Part print with two shaded views. Sizes in mm from the minimum x, y, z corner. A direction names the side the tool comes from. Round coordinates to 2 decimals unless told otherwise and drop trailing zeros. Loops run counter-clockwise (first coordinate to the right, second up) from the corner with the lowest first, then second, coordinate; pieces in that order, holes last. Notation, with made-up numbers: (-33, 73.25) - (8, 73.25) arc R25 cw to (8, 106.25) - close; hole circle Ø6 at (-30, 61). An arc over 180 degrees is marked (long way). Put each result on its own line as item: value. Start each with the question number.
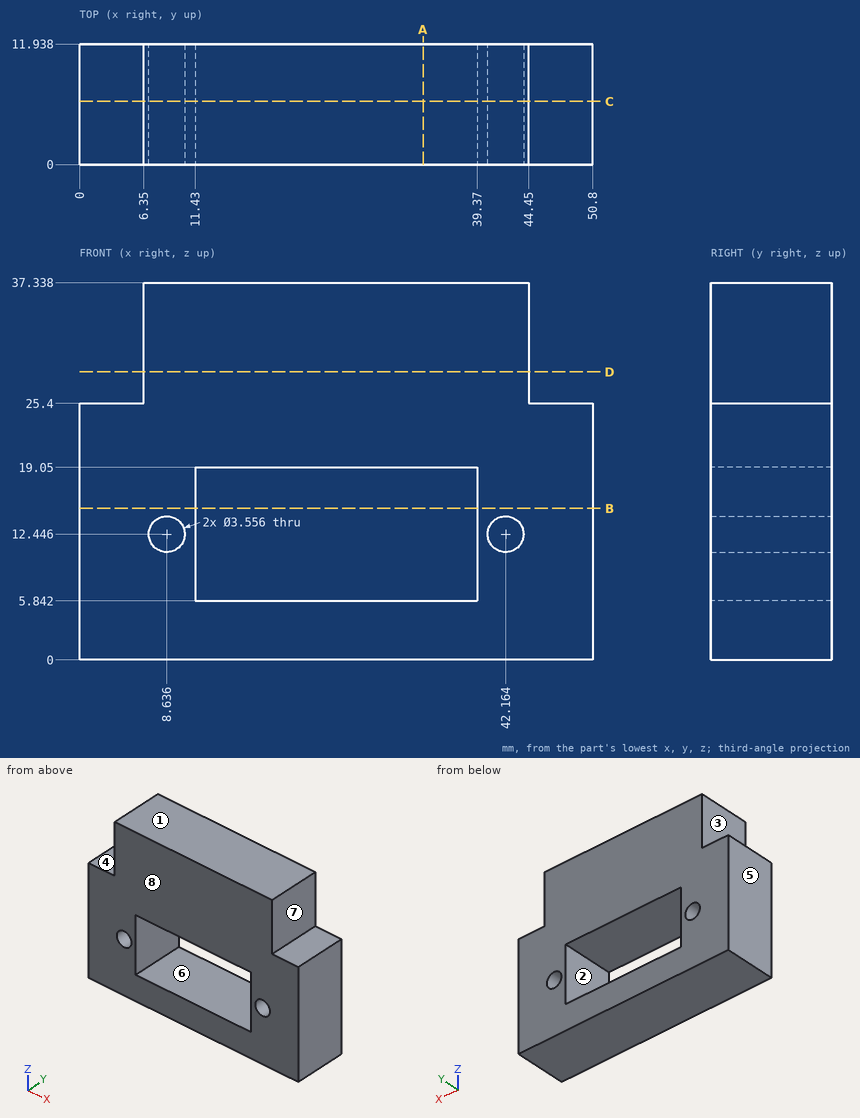
1) Slice it at A-A, the plane x = 34. Write the cut outline in (y, z).
2) Slice it at D-D, the plane z = 28.5. Write the cut outline in (x, y), and give its area (3 significant figures).
3) Pull direction X, two halves, no side cores. Call the marked faces 1, 2 and 3: pulls with the +X half, pulls with the -X half, needs draft (parallel to the pull), parting line crosses it, or undercut.
4) Drill centre lines: line 1 (X direction, y = 7.75, z = 6); line 2 (Z direction, x = 31, y = 2.75); line 3 (X direction, y = 4.5, z = 14). Where is each one in solid material? Low to high. Write a range as [from, to].
5) Slice it at C-C, the plane y = 6.25. Write the cut outline in (x, z), and give its area (3 significant figures).
6) Which spindle directions (+Z, -Z, +X, -X, +Y, -Y) get a long thin tool onto all of the face, cutting with end or side? Do the marked faces 4, 5, 6, 7 and 8. Say none if no direction does.
7) Drop flat-ended pins along their axis: pin 1 Ø1.9 at (x, y) = (48.5, 6.5) entering from +Z; pin 2 Ø6 at (y, z) = (9.5, 5) entering from -X; pin 3 Ø2 at (x, z) = (8.636, 12.446) entering from -Y; pin 4 Ø6 at (y, z) = (8.5, 33) entering from -X. Give the stop position or say it passes through.
8) Slice it at B-B, the plane z = 15. Write the cut outline in (x, y).
Taken from the geometry:
1. outline: (0, 0) - (11.94, 0) - (11.94, 5.84) - (0, 5.84) - close; (0, 19.05) - (11.94, 19.05) - (11.94, 37.34) - (0, 37.34) - close
2. outline: (6.35, 0) - (44.45, 0) - (44.45, 11.94) - (6.35, 11.94) - close
2. area: 455 mm2
3. face 1: needs draft
3. face 2: undercut
3. face 3: pulls with the -X half
4. line 1: x = [0, 11.43], [39.37, 50.8]
4. line 2: z = [0, 5.84], [19.05, 37.34]
4. line 3: x = [0, 7.77], [9.5, 11.43], [39.37, 41.3], [43.03, 50.8]
5. outline: (0, 0) - (50.8, 0) - (50.8, 25.4) - (44.45, 25.4) - (44.45, 37.34) - (6.35, 37.34) - (6.35, 25.4) - (0, 25.4) - close; hole circle Ø3.56 at (8.64, 12.45); hole (11.43, 5.84) - (39.37, 5.84) - (39.37, 19.05) - (11.43, 19.05) - close; hole circle Ø3.56 at (42.16, 12.45)
5. area: 1,360 mm2
6. face 4: +Z, -X, +Y, -Y
6. face 5: +Z, -Z, -X, +Y, -Y
6. face 6: +Y, -Y
6. face 7: +Z, +X, +Y, -Y
6. face 8: +Z, -Z, +X, -X, -Y
7. pin 1: stops at z = 25.4
7. pin 2: stops at x = 0
7. pin 3: passes through
7. pin 4: stops at x = 6.35
8. outline: (0, 0) - (11.43, 0) - (11.43, 11.94) - (0, 11.94) - close; (39.37, 0) - (50.8, 0) - (50.8, 11.94) - (39.37, 11.94) - close
